from build123d import *

# Parameters (mm, degrees)
SKETCH2_R           = 11.05
BOSS_EXTRUDE1_DEPTH = 3


with BuildPart() as part:
    # Sketch2 → Boss-Extrude1 (new body)
    with BuildSketch(Plane.XY.offset(777.361907162)):
        with BuildLine():
            Line((-21.864371204, -1.339746134), (-19.859932286, -34.051761818))
            Line((-19.859932286, -34.051761818), (23.868810121, -31.37226955))
            Line((23.868810121, -31.37226955), (21.864371204, 1.339746134))
            ThreePointArc((21.864371204, 1.339746134), (-1.339746134, 21.864371204), (-21.864371204, -1.339746134))
        make_face()
        Circle(SKETCH2_R, mode=Mode.SUBTRACT)
    extrude(amount=BOSS_EXTRUDE1_DEPTH)


solid = part.part
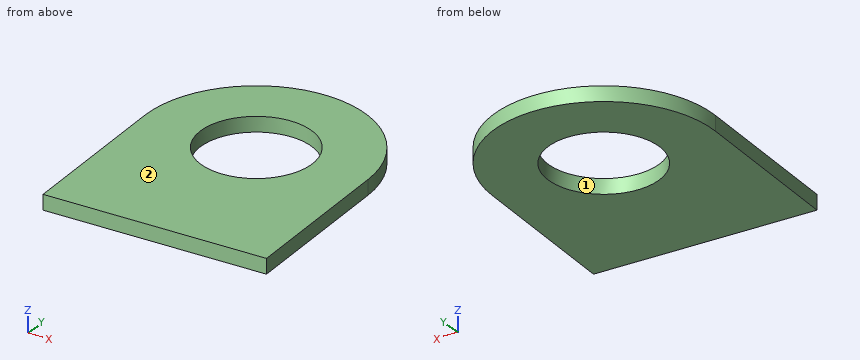
Source: CAD feature listing. Evaluate the final solid. Frame: model axes, mm. Face numbers are marked on the shaded views. Give positions to 0.01 mm unless a question says otherwise; leave off trailing zeros. Write each loop counter-clockwise with the first axis right and the second up, starting at its lowest first coordinate (ties: lowest second). Pieces come first, ordered by that corner, then holes. Notation, with made-up numbers: (79.5, 49.5) -> (128.5, 49.5) arc R24 ccw to (128.5, 85.5) -> close; hole circle Ø8 at (75, -33.5). An arc over 180 degrees is marked (long way). Return JSON: item names as keys, results as strings. Group by question number.
1. Section D-D, the plane y = 18. Output: boundary loops of the cut face in (x, z).
2. Mould query, pull axis X, two halves, no side actions, for the marked faces 1 and 2. Classes: +X half, -X half, draft (parallel to the pull), parting line (faces both ways), or undercut.
3. Pin query (flat end, axial travel): pin 1 Ø1.5 at (y, z) = (-5, 778) entering from +X; pin 2 Ø1 at (y, z) = (15.5, 778) entering from -X. Return the tip coordinate at first contact, or that it passes through.
4. Section C-C, the plane y = -8. Output: boundary loops of the cut face in (x, z), then the cut area to 3 significant figures.
5. Section B-B, the plane x = 0. Output: boundary loops of the cut face in (y, z), then the cut area to 3 significant figures.
6. Material intervals for line 1 (Y direction, x = 2.5, z = 778.55); line 2 (X direction, y = -1, z = 780.1); line 3 (Y direction, x = 0, z = 778.65), sorted ascending. Write a range as from..to.
Determined:
{
 "1": {"outline": "(-12.48, 777.36) -> (12.48, 777.36) -> (12.48, 780.36) -> (-12.48, 780.36) -> close"},
 "2": {"face 1": "undercut", "face 2": "draft"},
 "3": {"pin 1": "stops at x = 22.3", "pin 2": "stops at x = -15.96"},
 "4": {"outline": "(-21.46, 777.36) -> (-7.62, 777.36) -> (-7.62, 780.36) -> (-21.46, 780.36) -> close; (7.62, 777.36) -> (22.44, 777.36) -> (22.44, 780.36) -> (7.62, 780.36) -> close", "area": "85.9 mm2"},
 "5": {"outline": "(-32.83, 777.36) -> (-11.05, 777.36) -> (-11.05, 780.36) -> (-32.83, 780.36) -> close; (11.05, 777.36) -> (21.91, 777.36) -> (21.91, 780.36) -> (11.05, 780.36) -> close", "area": "97.9 mm2"},
 "6": {"line 1": "y = -32.68..-10.76, 10.76..21.76", "line 2": "x = -21.88..-11, 11..22.01", "line 3": "y = -32.83..-11.05, 11.05..21.91"}
}
